The listing builds one solid part. Answer for the finished solid, in the listing's coordinates (mm). A direction names the side the tool comes from. Round coordinates to 2 decimals unless told otherwise and drop trailing zeros. Order: outer loops, then holes, each group sorted by start corner. A loop starts at its lowest first (then second) coordinate and runs counter-clockwise, first axis right, second up. Notation, with made-up numbers: (57, -17) - (73, -17) arc R23 cw to (73, 20) - close; hole circle Ø7 at (58, -24). An arc over 180 degrees is marked (long way). One line per item, written item: value. Start each with the question number.
1. A tool of negligible diameter and unlimited length cuts with its end or side. For faces 5 (the flat face through (23.8, 11, 7.6)), 6 (the flat face through (6, -17, 11)), 7 (the flat face through (4, 0, 5.028)), 8 (the flat face through (-9, 17, 11)), from which of +Z, -Z, +X, -X, +Y, -Y can it reach the whole face along a straight path? Write none if from no direction.
2. Section C-C, the plane y = 10 is taken. Give the vertices of the cut face in (x, z).
3. Section D-D, the plane x = 15 is taken. Give the vertices of the cut face in (y, z), then the cut area to 3 significant figures.
4. Flat-ended cylindrical pins translate along their axes: P1, Ø2, axis at y = -10, z = 2.278, coming from the +X side; P2, Ø0.9, axis at x = -20.5, z = 3, coming from the -Y side; P3, Ø8, axis at x = -4, y = 8, coming from the +Z side; P4, Ø3, axis at x = 0.5, y = 6.5, coming from the -Z side. Find the tip coordinate at first contact, or state that the pin passes through.
5. Straight lines are drawn through the part: line 1 (Y direction, x = -6, z = 7); line 2 (Y direction, x = -15, z = 11.75); line 3 (Y direction, x = -3.5, z = 8.5). For each, find the intervals that lie inside material, in ascending order.
6. For a pull along X with two mould halves and no side action, classify faces 1 (the cylindrical face through (-20.887, -10.031, 3.528)), 2 (the cylindrical face through (15.176, -15.161, 8.725)), 3 (the flat face through (-24.25, 0, 7)), 4 (the flat face through (6, 17, 11)) as released by +X, released by -X, zero draft, split by the parting line, or undercut.
7. Section A-A, the plane x = -15 is taken. Give the vertices of the cut face in (y, z), then the cut area to 3 significant figures.
from build123d import *
from OCP.BRepFilletAPI import BRepFilletAPI_MakeChamfer

# Parameters (mm, degrees)
SKETCH_1_W                  = 48.5
SKETCH_1_H                  = 37
EXTRUDE_1_DEPTH             = 7.5
SKETCH_2_W                  = 4.5
SKETCH_2_H                  = 25
CUT_EXTRUDE_1_DEPTH         = 54.398977368
SKETCH_3_W                  = 41
SKETCH_3_H                  = 27.5
EXTRUDE_2_DEPTH             = 3.028
SKETCH_4_W                  = 38.25
SKETCH_4_H                  = 25
CUT_EXTRUDE_2_DEPTH         = 3.028
CUT_EXTRUDE_3_DEPTH         = 49.015109955
CUT_EXTRUDE_4_DEPTH         = 52.139033859
CUT_EXTRUDE_5_DEPTH         = 32.090983966
HOLE_WIZARD_2_5_2_5_1_D     = 2.5
HOLE_WIZARD_2_5_2_5_1_DEPTH = 1.75
HOLE_WIZARD_2_5_2_5_2_D     = 2.5
HOLE_WIZARD_2_5_2_5_2_DEPTH = 6
HOLE_WIZARD_2_5_2_5_3_D     = 2.5
HOLE_WIZARD_2_5_2_5_3_DEPTH = 4.25
HOLE_WIZARD_2_7_2_7_1_D     = 2.7
CHAMFER_1_SIZE              = 3
SKETCH_17_W                 = 3
SKETCH_17_H                 = 4
CUT_EXTRUDE_8_DEPTH         = 3
CHAMFER_2_SIZE              = 3
CHAMFER_2_SIZE_2            = 3.981134465
SKETCH_19_W                 = 2
SKETCH_19_H                 = 3
CUT_EXTRUDE_9_DEPTH         = 1.5
CHAMFER_3_SIZE              = 2
CHAMFER_4_SIZE              = 1
SKETCH_20_R                 = 3.2
CUT_EXTRUDE_10_DEPTH        = 21.5
SKETCH_21_W                 = 19.5
SKETCH_21_H                 = 15
CUT_EXTRUDE_11_DEPTH        = 21.5
CHAMFER_5_SIZE              = 2.5
SKETCH_22_W                 = 9
SKETCH_22_H                 = 15
CUT_EXTRUDE_12_DEPTH        = 51.5


# Some blends are built 0.0001 mm under size
with BuildPart() as part:
    # 草图1 → 凸台-拉伸1 (new body)
    with BuildSketch(Plane(origin=(0, 0, 5.028), x_dir=(-1, 0, 0), z_dir=(0, 0, -1))):
        Rectangle(SKETCH_1_W, SKETCH_1_H)
    extrude(amount=-EXTRUDE_1_DEPTH)

    # 草图2 → 切除-拉伸1 (cut, through all)
    with BuildSketch(Plane(origin=(24.25, 0, 0), x_dir=(0, 0, -1), z_dir=(1, 0, 0))):
        with Locations((-10.278, 0)):
            Rectangle(SKETCH_2_W, SKETCH_2_H)
    extrude(amount=-CUT_EXTRUDE_1_DEPTH, mode=Mode.SUBTRACT)

    # 草图3 → 凸台-拉伸2 (add)
    with BuildSketch(Plane(origin=(0, 0, 5.028), x_dir=(-1, 0, 0), z_dir=(0, 0, -1))):
        with Locations((1.25, 0)):
            Rectangle(SKETCH_3_W, SKETCH_3_H)
    extrude(amount=EXTRUDE_2_DEPTH)

    # 草图4 → 切除-拉伸2 (cut)
    with BuildSketch(Plane(origin=(0, 0, 2), x_dir=(-1, 0, 0), z_dir=(0, 0, -1))):
        with Locations((0.875, 0)):
            Rectangle(SKETCH_4_W, SKETCH_4_H)
    extrude(amount=-CUT_EXTRUDE_2_DEPTH, mode=Mode.SUBTRACT)

    # 草图5 → 切除-拉伸3 (cut, through all)
    with BuildSketch(Plane.ZY.offset(-18.25)):
        with BuildLine():
            Line((2, 7.034395212), (2, -7.034395212))
            ThreePointArc((2, -7.034395212), (4.278, 0), (2, 7.034395212))
        make_face()
    extrude(amount=-CUT_EXTRUDE_3_DEPTH, mode=Mode.SUBTRACT)

    # 草图6 → 切除-拉伸4 (cut, through all)
    with BuildSketch(Plane.ZY.offset(21.75)):
        with BuildLine():
            Line((2, 7.034395212), (2, -7.034395212))
            ThreePointArc((2, -7.034395212), (4.278, 0), (2, 7.034395212))
        make_face()
    extrude(amount=-CUT_EXTRUDE_4_DEPTH, mode=Mode.SUBTRACT)

    # 草图7 → 切除-拉伸5 (cut, through all)
    with BuildSketch(Plane.XY.offset(8.028)):
        with BuildLine():
            Line((-7.978419869, 7.029222073), (-13.021580131, 7.029222073))
            ThreePointArc((-13.021580131, 7.029222073), (-17.801221513, 4.934335949), (-19.5, 0))
            ThreePointArc((-19.5, 0), (-17.801221513, -4.934335949), (-13.021580131, -7.029222073))
            Line((-13.021580131, -7.029222073), (-7.978419869, -7.029222073))
            ThreePointArc((-7.978419869, -7.029222073), (-3.198778487, -4.934335949), (-1.5, 0))
            ThreePointArc((-1.5, 0), (-3.198778487, 4.934335949), (-7.978419869, 7.029222073))
        make_face()
    extrude(amount=-CUT_EXTRUDE_5_DEPTH, mode=Mode.SUBTRACT)

    # Ø2.5 (2.5) 直径孔1
    with Locations(Plane.ZY.offset(21.75)):
        with Locations((2.278, 10)):
            Hole(HOLE_WIZARD_2_5_2_5_1_D / 2, depth=HOLE_WIZARD_2_5_2_5_1_DEPTH)

    # Ø2.5 (2.5) 直径孔2
    with Locations(Plane.ZY.offset(-18.25)):
        with Locations((2.278, -10), (2.278, 10)):
            Hole(HOLE_WIZARD_2_5_2_5_2_D / 2, depth=HOLE_WIZARD_2_5_2_5_2_DEPTH)

    # Ø2.5 (2.5) 直径孔3
    with Locations(Plane(origin=(-20, 0, 0), x_dir=(0, 0, -1), z_dir=(1, 0, 0))):
        with Locations((-2.278, -10)):
            Hole(HOLE_WIZARD_2_5_2_5_3_D / 2, depth=HOLE_WIZARD_2_5_2_5_3_DEPTH)

    # Ø2.7 (2.7) 直径孔1 (through all)
    with Locations(Plane.XY.offset(12.528)):
        with Locations((0, -16.5), (-15, -16.5), (15, -16.5), (0, 16.5), (-15, 16.5), (15, 16.5)):
            Hole(HOLE_WIZARD_2_7_2_7_1_D / 2)

    # 倒角1
    chamfer_1_edges = [part.edges().sort_by_distance(p)[0] for p in [
        (-24.25, 18.5, 8.778),
        (-24.25, -18.5, 8.778),
        (24.25, -18.5, 8.778),
        (24.25, 18.5, 8.778),
    ]]
    chamfer(chamfer_1_edges, length=CHAMFER_1_SIZE)

    # 草图17 → 切除-拉伸8 (cut)
    with BuildSketch(Plane.XY.offset(12.528)):
        with Locations((-7.5, -16.5)):
            Rectangle(SKETCH_17_W, SKETCH_17_H)
        with Locations((7.5, -16.5)):
            Rectangle(SKETCH_17_W, SKETCH_17_H)
        with Locations((7.5, 16.5)):
            Rectangle(SKETCH_17_W, SKETCH_17_H)
        with Locations((-7.5, 16.5)):
            Rectangle(SKETCH_17_W, SKETCH_17_H)
    extrude(amount=-CUT_EXTRUDE_8_DEPTH, mode=Mode.SUBTRACT)

    # 倒角2
    chamfer_2_edges_1 = [part.edges().sort_by_distance(p)[0] for p in [
        (7.5, -14.5, 9.528),
    ]]
    chamfer_2_side_1 = [part.faces().sort_by_distance(p)[0] for p in [
        (7.5, -14.5, 9.588),
    ]]
    chamfer_2_edges_2 = [part.edges().sort_by_distance(p)[0] for p in [
        (-7.5, -14.5, 9.528),
    ]]
    chamfer_2_side_2 = [part.faces().sort_by_distance(p)[0] for p in [
        (-7.5, -14.5, 9.588),
    ]]
    chamfer_2_edges_3 = [part.edges().sort_by_distance(p)[0] for p in [
        (-7.5, 14.5, 9.528),
    ]]
    chamfer_2_side_3 = [part.faces().sort_by_distance(p)[0] for p in [
        (-7.5, 14.5, 9.588),
    ]]
    chamfer_2_edges_4 = [part.edges().sort_by_distance(p)[0] for p in [
        (7.5, 14.5, 9.528),
    ]]
    chamfer_2_side_4 = [part.faces().sort_by_distance(p)[0] for p in [
        (7.5, 14.5, 9.588),
    ]]
    chamfer_2 = BRepFilletAPI_MakeChamfer(part.part.solid().wrapped)
    for e in chamfer_2_edges_1:
        chamfer_2.Add(CHAMFER_2_SIZE - 0.0001, CHAMFER_2_SIZE_2 - 0.0001, e.wrapped, chamfer_2_side_1[0].wrapped)
    for e in chamfer_2_edges_2:
        chamfer_2.Add(CHAMFER_2_SIZE - 0.0001, CHAMFER_2_SIZE_2 - 0.0001, e.wrapped, chamfer_2_side_2[0].wrapped)
    for e in chamfer_2_edges_3:
        chamfer_2.Add(CHAMFER_2_SIZE - 0.0001, CHAMFER_2_SIZE_2 - 0.0001, e.wrapped, chamfer_2_side_3[0].wrapped)
    for e in chamfer_2_edges_4:
        chamfer_2.Add(CHAMFER_2_SIZE - 0.0001, CHAMFER_2_SIZE_2 - 0.0001, e.wrapped, chamfer_2_side_4[0].wrapped)
    add(Compound.cast(chamfer_2.Shape()), mode=Mode.REPLACE)  # a hair under: the kernel refuses the full size

    # 草图19 → 切除-拉伸9 (cut)
    with BuildSketch(Plane.XY.offset(8.028)):
        with Locations((-23.25, -9.5)):
            Rectangle(SKETCH_19_W, SKETCH_19_H)
        with Locations((-23.25, 9.5)):
            Rectangle(SKETCH_19_W, SKETCH_19_H)
        with Locations((23.25, 9.5)):
            Rectangle(SKETCH_19_W, SKETCH_19_H)
        with Locations((23.25, -9.5)):
            Rectangle(SKETCH_19_W, SKETCH_19_H)
    extrude(amount=-CUT_EXTRUDE_9_DEPTH, mode=Mode.SUBTRACT)

    # 倒角3
    # the kernel refuses this chamfer: 2 mm, written as the material it adds along each edge
    with BuildSketch(Plane(origin=(22.25, 11, 6.528), x_dir=(0.9996219169112968, 0, -0.02749587661058651), z_dir=(0, -1, 0))) as chamfer_3_piece_1_section:
        Polygon((CHAMFER_3_SIZE * 0.999621916911, CHAMFER_3_SIZE * 0.0274958766106), (-CHAMFER_3_SIZE * 0.0274958766106, CHAMFER_3_SIZE * 0.999621916911), (0, 0), align=None)
    chamfer_3_piece_1 = extrude(amount=8.143365976, mode=Mode.PRIVATE)
    chamfer_3_piece_1 = split(chamfer_3_piece_1, bisect_by=Plane(origin=(22.95, 9.5, 8.028), z_dir=(0, 0, -1)), keep=Keep.TOP, mode=Mode.PRIVATE)
    add(chamfer_3_piece_1)
    with BuildSketch(Plane(origin=(22.25, -11, 6.528), x_dir=(0.9996219169112968, 0, -0.02749587661058651), z_dir=(0, 1, 0))) as chamfer_3_piece_2_section:
        Polygon((CHAMFER_3_SIZE * 0.999621916911, -CHAMFER_3_SIZE * 0.0274958766106), (-CHAMFER_3_SIZE * 0.0274958766106, -CHAMFER_3_SIZE * 0.999621916911), (0, 0), align=None)
    chamfer_3_piece_2 = extrude(amount=8.143365976, mode=Mode.PRIVATE)
    chamfer_3_piece_2 = split(chamfer_3_piece_2, bisect_by=Plane(origin=(22.95, -9.5, 8.028), z_dir=(0, 0, -1)), keep=Keep.TOP, mode=Mode.PRIVATE)
    add(chamfer_3_piece_2)
    with BuildSketch(Plane(origin=(-22.25, 11, 6.528), x_dir=(-0.9996219169112968, 0, -0.02749587661058651), z_dir=(0, -1, 0))) as chamfer_3_piece_3_section:
        Polygon((CHAMFER_3_SIZE * 0.999621916911, -CHAMFER_3_SIZE * 0.0274958766106), (-CHAMFER_3_SIZE * 0.0274958766106, -CHAMFER_3_SIZE * 0.999621916911), (0, 0), align=None)
    chamfer_3_piece_3 = extrude(amount=8.143365976, mode=Mode.PRIVATE)
    chamfer_3_piece_3 = split(chamfer_3_piece_3, bisect_by=Plane(origin=(-22.95, 9.5, 8.028), z_dir=(0, 0, -1)), keep=Keep.TOP, mode=Mode.PRIVATE)
    add(chamfer_3_piece_3)
    with BuildSketch(Plane(origin=(-22.25, -16.143365976, 6.528), x_dir=(-0.9996219169112968, 0, -0.02749587661058651), z_dir=(0, 1, 0))) as chamfer_3_piece_4_section:
        Polygon((CHAMFER_3_SIZE * 0.999621916911, CHAMFER_3_SIZE * 0.0274958766106), (-CHAMFER_3_SIZE * 0.0274958766106, CHAMFER_3_SIZE * 0.999621916911), (0, 0), align=None)
    chamfer_3_piece_4 = extrude(amount=13.286731952, mode=Mode.PRIVATE)
    chamfer_3_piece_4 = split(chamfer_3_piece_4, bisect_by=Plane(origin=(-22.95, -9.5, 8.028), z_dir=(0, 0, -1)), keep=Keep.TOP, mode=Mode.PRIVATE)
    chamfer_3_piece_4 = split(chamfer_3_piece_4, bisect_by=Plane(origin=(-26.6, -13.15, 7.128), z_dir=(0.7071067811865476, 0.7071067811865476, 0)), keep=Keep.TOP, mode=Mode.PRIVATE)
    add(chamfer_3_piece_4)

    # 倒角4
    chamfer_4_edges = [part.edges().sort_by_distance(p)[0] for p in [
        (-21.75, 13.75, 3.514),
        (19.25, 13.75, 3.514),
        (19.25, -13.75, 3.514),
        (-21.75, -13.75, 3.514),
    ]]
    chamfer(chamfer_4_edges, length=CHAMFER_4_SIZE)

    # 草图20 → 切除-拉伸10 (cut)
    with BuildSketch(Plane(origin=(0, 0, 2), x_dir=(-1, 0, 0), z_dir=(0, 0, -1))):
        with Locations(Location((-10, 11.5, 0), (0, 0, 18.209956864))):
            Circle(SKETCH_20_R)
    extrude(amount=-CUT_EXTRUDE_10_DEPTH, mode=Mode.SUBTRACT)

    # 草图21 → 切除-拉伸11 (cut)
    with BuildSketch(Plane.XY.offset(8.028)):
        with Locations((-10, 0)):
            Rectangle(SKETCH_21_W, SKETCH_21_H)
    extrude(amount=-CUT_EXTRUDE_11_DEPTH, mode=Mode.SUBTRACT)

    # 倒角5
    chamfer_5_edges = [part.edges().sort_by_distance(p)[0] for p in [
        (-0.25, 7.5, 6.528),
        (-0.25, -7.5, 6.528),
        (-19.75, -7.5, 6.528),
        (-19.75, 7.5, 6.528),
    ]]
    chamfer(chamfer_5_edges, length=CHAMFER_5_SIZE)

    # 草图22 → 切除-拉伸12 (cut)
    with BuildSketch(Plane(origin=(19.25, 0, 0), x_dir=(0, 0, -1), z_dir=(1, 0, 0))):
        Rectangle(SKETCH_22_W, SKETCH_22_H)
    extrude(amount=-CUT_EXTRUDE_12_DEPTH, mode=Mode.SUBTRACT)


solid = part.part
Answer list:
1. face 5: +Z, +X
1. face 6: +Z, -Y
1. face 7: -Z
1. face 8: +Z, +Y
2. outline: (-24.25, 5.03) - (-21.75, 5.03) - (-21.75, 3.53) - (-20, 3.53) - (-20, 5.03) - (7.17, 5.03) - (7.17, 8.03) - (-22.75, 8.03) - (-24.25, 6.53) - close; (12.83, 5.03) - (18.25, 5.03) - (18.25, 3.53) - (19.25, 3.53) - (19.25, 5.03) - (24.25, 5.03) - (24.25, 6.53) - (22.75, 8.03) - (12.83, 8.03) - close
3. outline: (-18.5, 5.03) - (-17.85, 5.03) - (-17.85, 12.53) - (-18.5, 12.53) - close; (-15.15, 5.03) - (-13.75, 5.03) - (-13.75, 2) - (-12.5, 2) - (-12.5, 5.03) - (12.5, 5.03) - (12.5, 2) - (13.75, 2) - (13.75, 5.03) - (15.15, 5.03) - (15.15, 12.53) - (12.5, 12.53) - (12.5, 8.03) - (-12.5, 8.03) - (-12.5, 12.53) - (-15.15, 12.53) - close; (17.85, 5.03) - (18.5, 5.03) - (18.5, 12.53) - (17.85, 12.53) - close
3. area: 132 mm²
4. P1: passes through
4. P2: stops at y = -13.75
4. P3: stops at z = 8.03
4. P4: stops at z = 5.03
5. line 1: y = -18.5 to -7.5, 7.5 to 18.5
5. line 2: y = -18.5 to -17.85, -15.15 to -12.5, 12.5 to 15.15, 17.85 to 18.5
5. line 3: y = -18.5 to -12.5, 12.5 to 18.5
6. face 1: zero draft
6. face 2: undercut
6. face 3: released by -X
6. face 4: undercut
7. outline: (-18.5, 5.03) - (-17.85, 5.03) - (-17.85, 12.53) - (-18.5, 12.53) - close; (-15.15, 5.03) - (-13.75, 5.03) - (-13.75, 2) - (-12.5, 2) - (-12.5, 5.03) - (-7.5, 5.03) - (-7.5, 8.03) - (-12.5, 8.03) - (-12.5, 12.53) - (-15.15, 12.53) - close; (7.5, 5.03) - (12.5, 5.03) - (12.5, 2) - (13.75, 2) - (13.75, 5.03) - (15.15, 5.03) - (15.15, 12.53) - (12.5, 12.53) - (12.5, 8.03) - (7.5, 8.03) - close; (17.85, 5.03) - (18.5, 5.03) - (18.5, 12.53) - (17.85, 12.53) - close
7. area: 87.1 mm²
